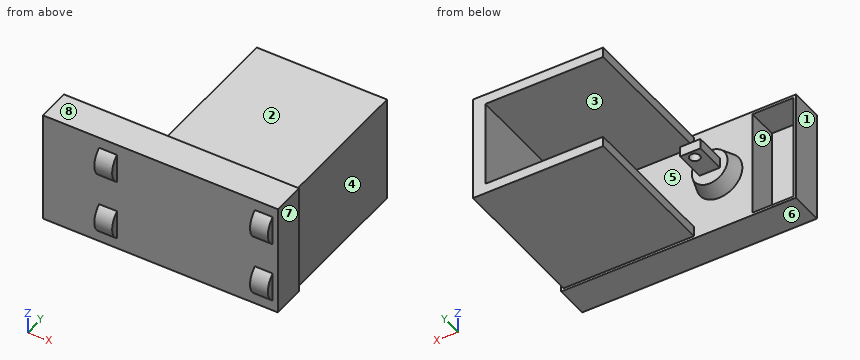
```python
from build123d import *

# Parameters (mm, degrees)
CHASIS_W                = 457.2
CHASIS_H                = 279.4
BOSS_EXTRUDE1_DEPTH     = 82.55
SKETCH3_W               = 44.45
SKETCH3_H               = 44.45
MIRROR2_COPY_1_SKETCH_W = 44.45
MIRROR2_COPY_1_SKETCH_H = 44.45
BOSS_EXTRUDE2_DEPTH     = 355.6
SKETCH6_R               = 44.45
SKETCH5_R               = 57.15
SKETCH10_W              = 279.4
SKETCH10_H              = 82.55
BOSS_EXTRUDE3_DEPTH     = 127
SKETCH11_W              = 101.6
SKETCH11_H              = 266.7
CUT_EXTRUDE1_DEPTH      = 76.2
SKETCH13_W              = 50.8
SKETCH13_H              = 25.4
BOSS_EXTRUDE5_DEPTH     = 76.2
SKETCH15_R              = 12.7
CUT_EXTRUDE2_DEPTH      = 25.4


with BuildPart() as part:
    # Chasis → Boss-Extrude1 (new body)
    with BuildSketch(Plane(origin=(0, 0, 0), x_dir=(1, 0, 0), z_dir=(0, 1, 0))):
        Rectangle(CHASIS_W, CHASIS_H)
    extrude(amount=BOSS_EXTRUDE1_DEPTH)

    # Sketch3 → Revolve1 (revolve)
    with BuildSketch(Plane(origin=(0, 25.4, 0), x_dir=(-1, 0, 0), z_dir=(0, -1, 0))):
        with Locations((193.675, -98.425)):
            Rectangle(SKETCH3_W, SKETCH3_H)
    revolve1 = revolve(axis=Axis((-215.9, 25.4, 76.2), (1, 0, 0)))

    # Mirror1: Revolve1 across plane
    add(revolve1.mirror(Plane.XY))

    # Mirror2: Revolve1 across plane
    add(revolve1.mirror(Plane(origin=(0, 0, 0), x_dir=(0, 0, 1), z_dir=(1, 0, 0))))

    # Mirror2 copy 1 sketch → Mirror2 copy 1 (revolve)
    with BuildSketch(Plane.XZ.offset(-25.4)):
        with Locations((193.675, -98.425)):
            Rectangle(MIRROR2_COPY_1_SKETCH_W, MIRROR2_COPY_1_SKETCH_H)
    revolve(axis=Axis((215.9, 25.4, -76.2), (-1, 0, 0)))

    # Sketch4 → Boss-Extrude2 (add)
    with BuildSketch(Plane(origin=(0, 82.55, 0), x_dir=(1, 0, 0), z_dir=(0, 1, 0))):
        Polygon((222.25, 133.35), (-101.6, 133.35), (-101.6, 107.95), (191.407142857, 107.95), (191.407142857, -107.95), (-101.6, -107.95), (-101.6, -133.35), (222.25, -133.35), align=None)
    extrude(amount=BOSS_EXTRUDE2_DEPTH)

    # Sketch6 → Loft1 section 0
    with BuildSketch(Plane(origin=(0, 120.65, 0), x_dir=(1, 0, 0), z_dir=(0, 1, 0))):
        with Locations((-165.1, 0)):
            Circle(SKETCH6_R)
    # Sketch5 → Loft1 section 1
    with BuildSketch(Plane(origin=(0, 82.55, 0), x_dir=(1, 0, 0), z_dir=(0, 1, 0))):
        with Locations((-165.1, 0)):
            Circle(SKETCH5_R)
    loft()

    # Sketch10 → Boss-Extrude3 (add)
    with BuildSketch(Plane.ZY.offset(228.6)):
        with Locations((0, 41.275)):
            Rectangle(SKETCH10_W, SKETCH10_H)
    extrude(amount=BOSS_EXTRUDE3_DEPTH)

    # Sketch11 → Cut-Extrude1 (cut)
    with BuildSketch(Plane(origin=(0, 82.55, 0), x_dir=(1, 0, 0), z_dir=(0, 1, 0))):
        with Locations((-298.45, 0)):
            Rectangle(SKETCH11_W, SKETCH11_H)
    extrude(amount=-CUT_EXTRUDE1_DEPTH, mode=Mode.SUBTRACT)

    # Sketch13 → Boss-Extrude5 (add)
    with BuildSketch(Plane(origin=(0, 120.65, 0), x_dir=(1, 0, 0), z_dir=(0, 1, 0))):
        with Locations((-165.1, 0)):
            Rectangle(SKETCH13_W, SKETCH13_H)
    extrude(amount=BOSS_EXTRUDE5_DEPTH)

    # Sketch15 → Cut-Extrude2 (cut)
    with BuildSketch(Plane.XY.offset(12.7)):
        with Locations((-164.332091847, 177.8)):
            Circle(SKETCH15_R)
    extrude(amount=-CUT_EXTRUDE2_DEPTH, mode=Mode.SUBTRACT)


solid = part.part
```
The listing builds one solid part. Answer for the finished solid, in the listing's coordinates (mm). Face numbers are marked on the shaded views. A direction names the side the tool comes from. Round coordinates to 2 decimals unless told otherwise and drop trailing zeros. Write each loop counter-clockwise with the first axis right and the second up, starting at its lowest first coordinate (ties: lowest second). Pieces come first, ordered by that corner, then holes. Notation, with made-up numbers: (-39, -33.75) -> (-21, -33.75) arc R26 cw to (-21, -2.75) -> close; hole circle Ø10 at (82.5, 40.5). An arc over 180 degrees is marked (long way). Answer as a JSON object with one key per item and string values. Group by question number.
Q1. Determine the mould class of the marked faces 6, 7, 8 and 9 for opening direction Z: pulls with the +Z half, pulls with the -Z half, needs draft (parallel to the pull), parting line crosses it, or undercut.
Q2. Section B-B (y = 177.8) is taken. Write down the section's boundary in (x, z), plus the area to 3 significant figures.
Q3. Each of these flat-tipped pins is pushed along its axis until it touches: pin 1 Ø12.5 at (y, z) = (167, 1) entering from +X; pin 2 Ø9.5 at (y, z) = (-11.5, -79) entering from +X; pin 3 Ø20.5 at (y, z) = (177.5, 123) entering from -X. Where does it stop, or does it pass through?
Q4. Section C-C (x = -64) is taken. Write down the section's boundary in (y, z).
Q5. Section A-A (y = 107) is taken. Write down the section's boundary in (x, z), plus the area to 3 significant figures.
Q6. Section D-D (x = -165.1) is taken. Write down the section's boundary in (y, z).
Q7. Straight lines are drawn through the part: line 1 along X through (y, z) = (177, -5); line 2 along Z through (x, y) = (-39, 401.5); line 3 along X through (y, z) = (32.5, -9). For each, find the intervals that lie inside material, in ascending order.
Q8. Which of the six approach directions +Z, -Z, +X, -X, +Y, -Y give full straight-line access (tool end or side, diameter ignored) to the marked faces 1, 2, 3, 4 and 5?
Check values:
{
 "1": {"face 6": "pulls with the -Z half", "face 7": "needs draft", "face 8": "pulls with the +Z half", "face 9": "undercut"},
 "2": {"outline": "(-190.5, -12.7) -> (-177.03, -12.7) -> (-177.03, 12.7) -> (-190.5, 12.7) -> close; (-151.63, -12.7) -> (-139.7, -12.7) -> (-139.7, 12.7) -> (-151.63, 12.7) -> close; (-101.6, -133.35) -> (222.25, -133.35) -> (222.25, 133.35) -> (-101.6, 133.35) -> (-101.6, 107.95) -> (191.41, 107.95) -> (191.41, -107.95) -> (-101.6, -107.95) -> close", "area": "23,800 mm^2"},
 "3": {"pin 1": "x = 222.25", "pin 2": "x = 215.9", "pin 3": "x = -101.6"},
 "4": {"outline": "(0, -139.7) -> (82.55, -139.7) -> (82.55, -133.35) -> (438.15, -133.35) -> (438.15, -107.95) -> (82.55, -107.95) -> (82.55, 107.95) -> (438.15, 107.95) -> (438.15, 133.35) -> (82.55, 133.35) -> (82.55, 139.7) -> (0, 139.7) -> close"},
 "5": {"outline": "circle Ø98 at (-165.1, 0); (-101.6, -133.35) -> (222.25, -133.35) -> (222.25, 133.35) -> (-101.6, 133.35) -> (-101.6, 107.95) -> (191.41, 107.95) -> (191.41, -107.95) -> (-101.6, -107.95) -> close", "area": "30,700 mm^2"},
 "6": {"outline": "(0, -139.7) -> (82.55, -139.7) -> (82.55, -57.15) -> (120.65, -44.45) -> (120.65, -12.7) -> (165.12, -12.7) -> (165.12, 12.7) -> (120.65, 12.7) -> (120.65, 44.45) -> (82.55, 57.15) -> (82.55, 139.7) -> (0, 139.7) -> close; (190.48, -12.7) -> (196.85, -12.7) -> (196.85, 12.7) -> (190.48, 12.7) -> close"},
 "7": {"line 1": "-190.5 to -177.01, -151.66 to -139.7, 191.41 to 222.25", "line 2": "-133.35 to -107.95, 107.95 to 133.35", "line 3": "-355.6 to -349.25, -247.65 to 228.6"},
 "8": {"face 1": "+Z, -Z, -X, +Y, -Y", "face 2": "+Z, +X, -X, +Y", "face 3": "-X, +Y", "face 4": "+Z, -Z, +X, +Y", "face 5": "+Y"}
}
